Print and shaded views of the part. All mm, measured from the part's lowest x, y and z. A direction names the side the tool comes from. Round coordinates to 2 decimals unless told otherwise and drop trailing zeros. Loops run counter-clockwise (first coordinate to the right, second up) from the corner with the lowest first, then second, coordinate; pieces in that order, holes last. Notation, with made-up numbers: (-22, 26) - (30, 26) arc R13 cw to (30, 47) - close; hole circle Ø1 at (-29, 82.25). An arc over 180 degrees is marked (long way). Use one line per item in the form item = value. Start each with the question number.
Q1. 3-axis set-ups, long thin cutter, end or side, ignore diameter. For the marked faces 1 and 2: which of +Z, -Z, +X, -X, +Y, -Y reach the whole face in a straight line?
Q2. Drill centre lines: line 1 (Z direction, x = 47.5, y = 1.45); line 2 (Z direction, x = 5, y = 35); line 3 (X direction, y = 55, z = 76). Where is each one in solid material? Low to high.
Q3. Pin check, flat tips, straight feed: pin 1 (8 mm diameter, centred on x = 70, y = 29.5, fed in from -Z); pin 2 (5 mm diameter, centred on x = 14, z = 26, fed in from +Y). Stop position of each tip, or through.
Q4. Saw through at C-C (x = 40). Give the cut face in (y, z).
Q5. Saw through at A-A (y = 38.5). Give the cut face in (x, z).
Q6. Saw through at D-D (y = 55). Give the cut face in (x, z).
Q7. Mould opens along Z. For the marked faces 3, 4 and 5 say: released by +Z, released by -Z, zero draft, split by the parting line, or undercut.
Q8. Saw through at B-B (z = 67.5). Give the cut face in (x, y).
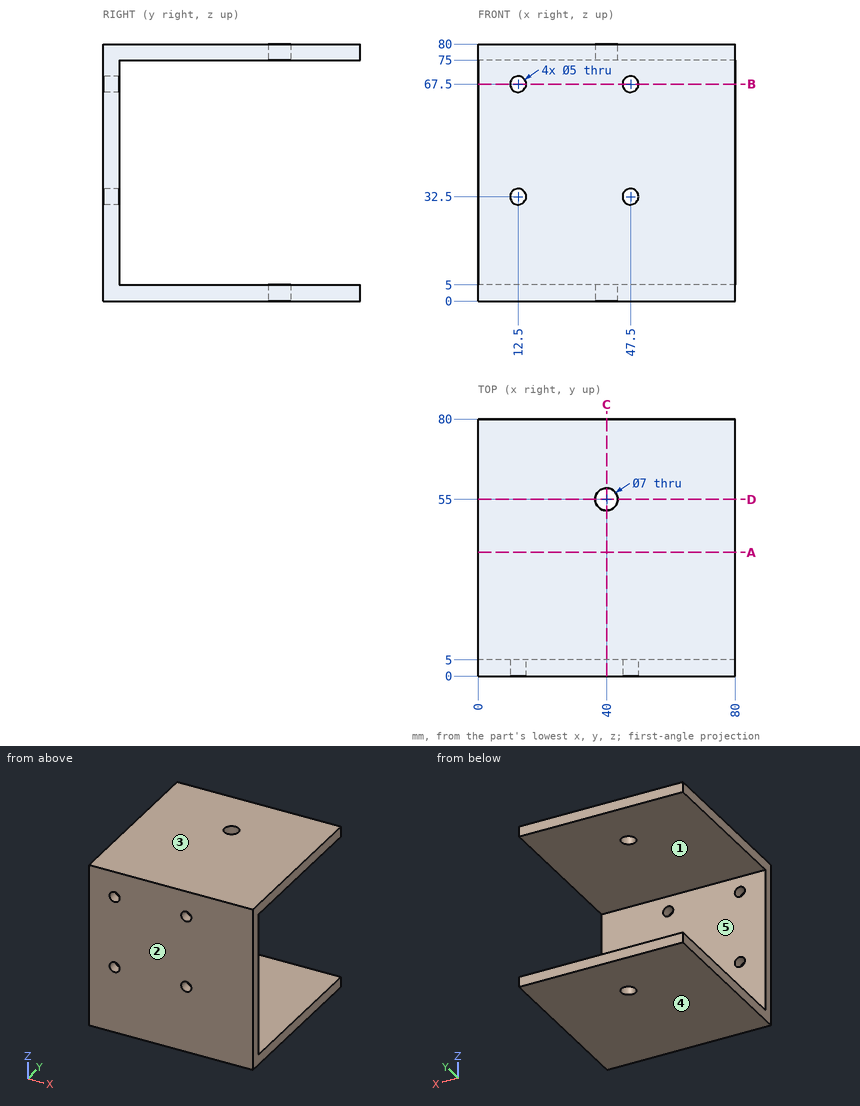
Report:
q1.face_1 = +X, -X, +Y
q1.face_2 = +Z, -Z, +X, -X, -Y
q2.line_1 = 0 to 30, 35 to 65, 70 to 80
q2.line_2 = 0 to 5, 75 to 80
q2.line_3 = 0 to 36.5, 43.5 to 80
q3.pin_1 = 0
q3.pin_2 = 5
q4.outline = (0, 0) - (51.5, 0) - (51.5, 5) - (5, 5) - (5, 75) - (51.5, 75) - (51.5, 80) - (0, 80) - close; (58.5, 0) - (80, 0) - (80, 5) - (58.5, 5) - close; (58.5, 75) - (80, 75) - (80, 80) - (58.5, 80) - close
q5.outline = (0, 0) - (80, 0) - (80, 5) - (0, 5) - close; (0, 75) - (80, 75) - (80, 80) - (0, 80) - close
q6.outline = (0, 0) - (36.5, 0) - (36.5, 5) - (0, 5) - close; (0, 75) - (36.5, 75) - (36.5, 80) - (0, 80) - close; (43.5, 0) - (80, 0) - (80, 5) - (43.5, 5) - close; (43.5, 75) - (80, 75) - (80, 80) - (43.5, 80) - close
q7.face_3 = released by +Z
q7.face_4 = released by -Z
q7.face_5 = undercut
q8.outline = (0, 0) - (10, 0) - (10, 5) - (0, 5) - close; (15, 0) - (45, 0) - (45, 5) - (15, 5) - close; (50, 0) - (80, 0) - (80, 5) - (50, 5) - close
